Read the model definition and answer for the solid it produces. Units are mm, in the model's axes. A direction names the side the tool comes from. Give positions to 0.01 mm unless a question says otherwise; leave off trailing zeros. Write each loop counter-clockwise with the first axis right and the second up, starting at its lowest first coordinate (ties: lowest second). Pieces come first, ordered by that corner, then holes. Notation, with made-up numbers: M 37,23 L 93,23 A18 cw 93,50 Z; hole C 61.5,-15.75 d1. An arc over 180 degrees is marked long. Write each question's results on one line, items separated by ' | '. Start each with the question number.
```python
from build123d import *

# Parameters (mm, degrees)
F0_R       = 1.4
F1_DEPTH   = 2
F2_W       = 4.8
F2_H       = 6
F3_DEPTH   = 2
F4_SIZE2   = 1.5
F4_SIZE    = 0.75
F4_2_SIZE2 = 1.5
F4_2_SIZE  = 0.75
F5_R       = 1
F7_DEPTH   = 4.001
F8_SIZE2   = 1
F8_SIZE    = 0.5
F9_R       = 2.5


with BuildPart() as f1:
    # F0 (on Top) → F1 (new body, symmetric)
    with BuildSketch(Plane.XY):
        with BuildLine():
            ThreePointArc((3.5, -4.3301270189), (3.610177635, -3.6754733482), (3.9285714286, -3.0929478707))
            ThreePointArc((3.9285714286, -3.0929478707), (0, 5), (-3.9285714286, -3.0929478707))
            ThreePointArc((-3.9285714286, -3.0929478707), (-3.610177635, -3.6754733482), (-3.5, -4.3301270189))
            Line((-3.5, -4.3301270189), (-3.5, -5.75))
            ThreePointArc((-3.5, -5.75), (-3.2071067812, -6.4571067812), (-2.5, -6.75))
            Line((-2.5, -6.75), (2.5, -6.75))
            ThreePointArc((2.5, -6.75), (3.2071067812, -6.4571067812), (3.5, -5.75))
            Line((3.5, -5.75), (3.5, -4.3301270189))
        make_face()
        with BuildLine():
            ThreePointArc((0.8227241336, -2.725), (0.8227241336, -2.975), (0.6062177826, -3.1))
            Line((0.6062177826, -3.1), (-0.6062177826, -3.1))
            ThreePointArc((-0.6062177826, -3.1), (-0.8227241336, -2.975), (-0.8227241336, -2.725))
            Line((-0.8227241336, -2.725), (-0.2165063509, -1.675))
            ThreePointArc((-0.2165063509, -1.675), (0, -1.55), (0.2165063509, -1.675))
            Line((0.2165063509, -1.675), (0.8227241336, -2.725))
        make_face(mode=Mode.SUBTRACT)
        with Locations((-2, -0.2)):
            Circle(F0_R, mode=Mode.SUBTRACT)
        with Locations((2, -0.2)):
            Circle(F0_R, mode=Mode.SUBTRACT)
    extrude(amount=F1_DEPTH, both=True)

    # F2 (on Top) → F3 (join, symmetric)
    with BuildSketch(Plane.XY):
        with Locations((0, -8)):
            Rectangle(F2_W, F2_H)
    extrude(amount=F3_DEPTH, both=True)

    # F4
    f4_edges = [f1.edges().sort_by_distance(p)[0] for p in [
        (2.4, -8.875, 2),
        (-2.4, -8.875, 2),
    ]]
    f4_side = f1.faces().sort_by_distance((3.07369, -6.32369, 2))[0]
    chamfer(f4_edges, length=F4_SIZE, length2=F4_SIZE2, reference=f4_side)

    # F4#2
    f4_2_edges = [f1.edges().sort_by_distance(p)[0] for p in [
        (2.4, -8.875, -2),
        (-2.4, -8.875, -2),
    ]]
    f4_2_side = f1.faces().sort_by_distance((3.07369, -6.32369, -2))[0]
    chamfer(f4_2_edges, length=F4_2_SIZE, length2=F4_2_SIZE2, reference=f4_2_side)

    # F5
    f5_edges = [f1.edges().sort_by_distance(p)[0] for p in [
        (2.4, -8.875, 0.5),
        (2.4, -8.875, -0.5),
        (-2.4, -8.875, 0.5),
        (-2.4, -8.875, -0.5),
    ]]
    fillet(f5_edges, radius=F5_R)

    # F6 (on face) → F7 (cut, through all)
    with BuildSketch(Plane.XY.offset(2)):
        with BuildLine():
            ThreePointArc((-2.15, -5.5), (-1.75, -5.9), (-1.35, -5.5))
            Line((-1.35, -5.5), (-1.35, -4.5))
            ThreePointArc((-1.35, -4.5), (-1.75, -4.1), (-2.15, -4.5))
            Line((-2.15, -4.5), (-2.15, -5.5))
        make_face()
        with BuildLine():
            ThreePointArc((0.4, -4.5), (0, -4.1), (-0.4, -4.5))
            Line((-0.4, -4.5), (-0.4, -5.5))
            ThreePointArc((-0.4, -5.5), (0, -5.9), (0.4, -5.5))
            Line((0.4, -5.5), (0.4, -4.5))
        make_face()
        with BuildLine():
            ThreePointArc((2.15, -4.5), (1.75, -4.1), (1.35, -4.5))
            Line((1.35, -4.5), (1.35, -5.5))
            ThreePointArc((1.35, -5.5), (1.75, -5.9), (2.15, -5.5))
            Line((2.15, -5.5), (2.15, -4.5))
        make_face()
    extrude(amount=-F7_DEPTH, mode=Mode.SUBTRACT)

    # F8
    f8_edges = [f1.edges().sort_by_distance(p)[0] for p in [
        (1.972214, -11, -1.355573),
        (2.373249, -11, -0.493685),
        (2.4, -11, 0),
        (2.373249, -11, 0.493685),
        (1.972214, -11, 1.355573),
        (-1.972214, -11, 1.355573),
    ]]
    chamfer(f8_edges, length=F8_SIZE, length2=F8_SIZE2)

    # F9
    f9_edges = [f1.edges().sort_by_distance(p)[0] for p in [
        (1.972214, -10, 1.355573),
        (-1.972214, -10, 1.355573),
    ]]
    fillet(f9_edges, radius=F9_R)


solid = f1.part
```
Item 1: Section A-A, the plane x = 0 is taken. Determine the outline of the cut face in (y, z), then the cut area to 3 significant figures.
Item 2: Determine the mould class of faces 1 (the cylindrical face through (0, -5.9, 0)), 2 (the cylindrical face through (0.6, -0.14, -0.03)), 3 (the flat face through (2, -8.1, -1.3)), 4 (the cylindrical face through (1.89, -9.99, -1.37)) for opening direction Y: +Y half, -Y half, draft (parallel to the pull), parting line (faces both ways), or undercut.
Item 3: Section D-D, the plane x = 2.75 is taken. Determine the outline of the cut face in (y, z).
Item 4: Section C-C, the plane y = 0.5 is taken. Determine the outline of the cut face in (x, z).
Item 5: Section B-B, the plane y = -7.75 is taken. Determine the outline of the cut face in (x, z).
Item 6: Straight lines are drawn through the part: line 1 (X direction, y = 0.75, z = -1.35); line 2 (Y direction, x = -2, z = 0); line 3 (Y direction, x = -2, z = -1.7). For each, find the intervals that lie inside material, in ascending order.
Item 7: For faces 5 (the cylindrical face through (1.88, -9.99, 1.39)), 6 (the flat face through (-2.15, -5, 0)), determine the directions among +Z, -Z, +X, -X, +Y, -Y from which every point of the face is accessible in a straight line to the end or side of a thin tool.
Item 8: Given P1, Ø1.1, axis at y = -5, z = -0.5, coming from the +X side; P2, Ø1.6, axis at y = -5, z = -1, coming from the -X side; P3, Ø0.6, axis at y = -8.5, z = 0, coming from the +X side, each flat-ended and moving along its own axis, determine where each tip first touches the part or whether it passes through.
Worked out:
1) outline: M -11,-2 L -5.9,-2 L -5.9,2 L -11,2 Z; M -4.1,-2 L -3.1,-2 L -3.1,2 L -4.1,2 Z; M -1.55,-2 L 5,-2 L 5,2 L -1.55,2 Z | area: 50.6 mm²
2) face 1: undercut | face 2: undercut | face 3: draft | face 4: -Y half
3) outline: M -6.72,-2 L -1.38,-2 L -1.38,2 L -6.72,2 Z; M 0.98,-2 L 4.18,-2 L 4.18,2 L 0.98,2 Z
4) outline: M -4.97,-2 L -3.21,-2 L -3.21,2 L -4.97,2 Z; M -0.79,-2 L 0.79,-2 L 0.79,2 L -0.79,2 Z; M 3.21,-2 L 4.97,-2 L 4.97,2 L 3.21,2 Z
5) outline: M -2.4,-0.26 A1 ccw -2.29,-0.71 L -1.65,-2 L 1.65,-2 L 2.29,-0.71 A1 ccw 2.4,-0.26 L 2.4,0.26 A1 ccw 2.29,0.71 L 1.65,2 L -1.65,2 L -2.29,0.71 A1 ccw -2.4,0.26 Z
6) line 1: x = -4.94 to -3.03, -0.97 to 0.97, 3.03 to 4.94 | line 2: y = -10.8 to -5.81, -4.19 to -1.6, 1.2 to 4.58 | line 3: y = -6.75 to -5.81, -4.19 to -1.6, 1.2 to 4.58
7) face 5: +Z, +X, -Y | face 6: +Z, -Z
8) P1: stops at x = 3.5 | P2: stops at x = -3.5 | P3: stops at x = 2.4
